Autodesk Inventor part; units mm, degrees
sketch "Sketch1" plane through (0, 0, 0) normal (0, 0, 1) x (1, 0, 0)
  circle A0 centre (-49.8513, 0) radius 7.5
  circle A1 centre (50.2519, 0) radius 7.5
  line L0 (-57.7949, 20.5158) -> (-14.443, 37.3015)
  arc A2 (-57.7949, 20.5158) -> (-57.7949, -20.5158) centre (-49.8513, 0) ccw
  arc A3 (58.1322, -20.5402) -> (58.1322, 20.5402) centre (50.2519, 0) ccw
  line L1 (14.3278, 37.3459) -> (58.1322, 20.5402)
  line L2 (58.1322, -20.5402) -> (14.3278, -37.3459)
  line L3 (-57.7949, -20.5158) -> (-14.443, -37.3015)
  arc A4 (-14.443, -37.3015) -> (14.3278, -37.3459) centre (0, 0) ccw
  arc A5 (14.3278, 37.3459) -> (-14.443, 37.3015) centre (0, 0) ccw
  dimension "d19" = 15
  dimension "d20" = 15
  dimension "d45" = 44
  dimension "d46" = 44
  dimension "d47" = 0
  dimension "d48" = 0
sketch "Sketch2" plane through (0, 0, 0) normal (1, 0, 0) x (0, 1, 0)
  line L0 (-20.5849, 0) -> (20.5849, 0)
  line L1 (20.5849, 0) -> (20.5849, 18)
  line L2 (-20.5849, 18) -> (-20.5849, 18)
  line L3 (-20.5849, 0) -> (-20.5849, 18)
  line L4 (-20.5849, 18) -> (-20.5849, 18)
  line L5 (-33.5, 18) -> (33.5, 18)
  line L6 (33.5, 18) -> (22.6557, 79.9649)
  line L7 (-22.6557, 79.9649) -> (-33.5, 18)
  circle A0 centre (0, 76) radius 23
  circle A1 centre (0, 76) radius 15
  point P0 (0, 0)
  dimension "d23" = 67
  dimension "d25" = 0
  dimension "d27" = 33.5
  dimension "d37" = 30
  dimension "d38" = 46
  dimension "d39" = 58
extrude "Extrusion5" add sketch "Sketch2" along normal mid plane 18 contours L5 L7 A0 L6
extrude "Extrusion6" add sketch "Sketch2" along normal mid plane 40 contours A0
extrude "Extrusion7" add sketch "Sketch1" along normal blind 18
properties part number "6.2_DATE11_1"
Check sheet for the modelled part. Datum: model origin and axes. Units: mm. A direction names the side the tool comes from. Coordinates: 2 decimals unless noted, no trailing zeros. Loops run counter-clockwise (first coordinate to the right, second up) from the corner with the lowest first, then second, coordinate; pieces in that order, holes last.
1) Release check for a two-part mould opening along Y. For faces 6 (the face through (0, 40, 9)), 7 (the face through (57.406, -2.253, 8.874)), 8 (the face through (0, -40, 9)) record: released by +Y, released by -Y, zero draft, split by the parting line, or undercut.
2) Sectioned sample at D-D (y = -11). Record the boundary of the cut face in (x, z).
3) Material ranges on probe 1 along Z at (x, y) = (-6, 0); probe 2 along Z at (x, y) = (-12.5, -11.5); probe 3 along X at (y, z) = (21.5, 47), recorded low to high.
4) Sectioned sample at B-B (y = 0). Record the boundary of the cut face in (x, z).
5) Sectioned sample at A-A (z = 15.5). Record the boundary of the cut face in (x, y).
6) Gauge pin test, flat ends, axial feed: pin 1 (12 mm diameter, centred on y = 30, z = 52, fed in from +X); pin 2 (17 mm diameter, centred on x = -49.85, y = 0, fed in from +Z); pin 3 (12 mm diameter, centred on x = 50.25, y = 0, fed in from +Z); pin 4 (23 mm diameter, centred on y = 2.5, z = 80.5, fed in from +X). Record the tip position at first contact, or that the pin passes through.
7) Access from +Z, -Z, +X, -X, +Y, -Y to the whole of each face (thin tool, end or side, straight path). Record for faces 1 (the face through (-71.85, -0.37, 8.87)), 2 (the face through (-0.28, 10.613, 96.405)), 3 (the face through (-42.698, -2.253, 8.874)), 4 (the face through (-20, 5, 61)), 5 (the face through (20, 5, 61)).
8) Sectioned sample at C-C (x = 12). Record the boundary of the cut face in (y, z), and give its area (3 significant figures).
Check sheet entries:
1. face 6: released by +Y
1. face 7: undercut
1. face 8: released by -Y
2. outline: (-68.9, 0) - (69.3, 0) - (69.3, 18) - (9, 18) - (9, 55.8) - (20, 55.8) - (20, 65.8) - (-20, 65.8) - (-20, 55.8) - (-9, 55.8) - (-9, 18) - (-68.9, 18) - close; (-20, 86.2) - (20, 86.2) - (20, 96.2) - (-20, 96.2) - close
3. probe 1: z = 0 to 61, 91 to 99
3. probe 2: z = 0 to 18, 56.08 to 66.37, 85.63 to 95.92
3. probe 3: x = -9 to 9
4. outline: (-71.85, 0) - (-57.35, 0) - (-57.35, 18) - (-71.85, 18) - close; (-42.35, 0) - (42.75, 0) - (42.75, 18) - (9, 18) - (9, 53) - (20, 53) - (20, 61) - (-20, 61) - (-20, 53) - (-9, 53) - (-9, 18) - (-42.35, 18) - close; (-20, 91) - (20, 91) - (20, 99) - (-20, 99) - close; (57.75, 0) - (72.25, 0) - (72.25, 18) - (57.75, 18) - close
5. outline: (-57.79, -20.52) - (-14.44, -37.3) arc R40 ccw to (14.33, -37.35) - (58.13, -20.54) arc R22 ccw to (58.13, 20.54) - (14.33, 37.35) arc R40 ccw to (-14.44, 37.3) - (-57.79, 20.52) arc R22 ccw to start; hole circle Ø15 at (-49.85, 0); hole circle Ø15 at (50.25, 0)
6. pin 1: stops at x = 9
6. pin 2: stops at z = 18
6. pin 3: passes through
6. pin 4: stops at x = 20
7. face 1: +Z, -Z, -X
7. face 2: none
7. face 3: +Z, -Z
7. face 4: +Z, -X, +Y, -Y
7. face 5: +Z, +X, +Y, -Y
8. outline: (-38.16, 0) - (38.16, 0) - (38.16, 18) - (-38.16, 18) - close; circle Ø46 at (0, 76); hole circle Ø30 at (0, 76)
8. area: 2,330 mm2
